The figure shows three views and two pictorial views of one solid part (mm, origin at its lowest corner). Answer the questions. A direction names the side the tool comes from. Give positions to 0.01 mm unless a question says otherwise; leave off trailing zeros. Loops run counter-clockwise (first coordinate to the right, second up) from the corner with the lowest first, then second, coordinate; pieces in that order, holes last. Notation, with made-up numbers: (-22.5, 40.5) -> (-1.5, 40.5) arc R12 cw to (-1.5, 59.5) -> close; hole circle Ø6 at (-25, 47.5). An arc over 180 degrees is marked (long way). Answer as CSV lines item,"result". Start each with the question number.
1. Find section A-A, the plane x = 640.5. Give the vertices of the cut face in (y, z).
2. A tool of negligible diameter and unlimited length cuts with its end or side. For the marked faces 5 and 6, from which of +Z, -Z, +X, -X, +Y, -Y can it reach the whole face along a straight path? Write none if from no direction.
3. Find the intervals of material crossed by line 1 along X through (y, z) = (230.5, 17.5); line 2 along Y through (x, z) = (627, 41); line 3 along Y through (x, z) = (240, 242.5), in increasing order.
4. Determine the mould class of the marked faces 1, 2, 3 and 4 for opening direction Y: +Y half, -Y half, draft (parallel to the pull), parting line (faces both ways), or undercut.
5. Find section B-B, the plane y = 400.05. Give the vertices of the cut face in (x, z), and give its area (3 significant figures).
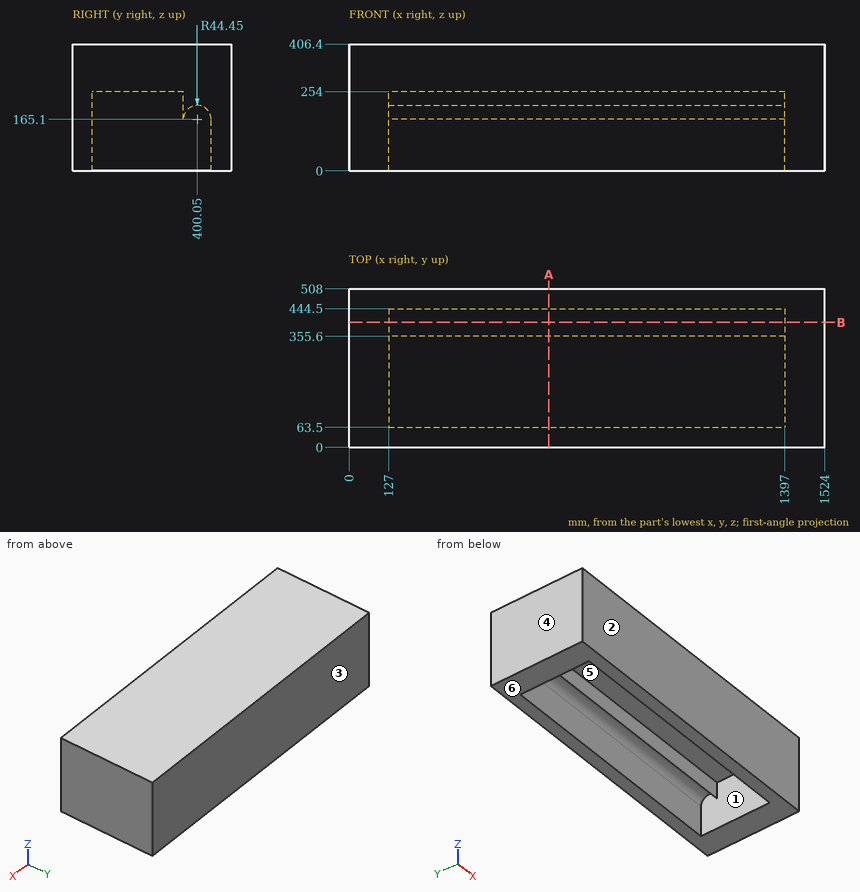
Resolved:
1,outline,"(0, 0) -> (63.5, 0) -> (63.5, 254) -> (355.6, 254) -> (355.6, 165.1) arc R44.45 cw to (444.5, 165.1) -> (444.5, 0) -> (508, 0) -> (508, 406.4) -> (0, 406.4) -> close"
2,face 5,"-Z"
2,face 6,"-Z, +X, -X, +Y, -Y"
3,line 1,"x = 0 to 127, 1397 to 1524"
3,line 2,"y = 0 to 63.5, 444.5 to 508"
3,line 3,"y = 0 to 63.5, 355.6 to 508"
4,face 1,"undercut"
4,face 2,"-Y half"
4,face 3,"+Y half"
4,face 4,"draft"
5,outline,"(0, 0) -> (127, 0) -> (127, 209.55) -> (1397, 209.55) -> (1397, 0) -> (1524, 0) -> (1524, 406.4) -> (0, 406.4) -> close"
5,area,"353,000 mm^2"
